For this review, take the finished solid that the model builds, in its own axes (mm). Face numbers are marked on the shaded views. A direction names the side the tool comes from. Give positions to 0.01 mm unless a question says otherwise; leave off trailing zeros. Loops run counter-clockwise (first coordinate to the right, second up) from the corner with the lowest first, then second, coordinate; pieces in that order, holes last. Notation, with made-up numbers: (35.5, -12) - (46.5, -12) arc R10 ccw to (46.5, -1) - close; hole circle Ø5 at (-25, -28). An arc over 180 degrees is marked (long way). Put each result on its own line as item: value.
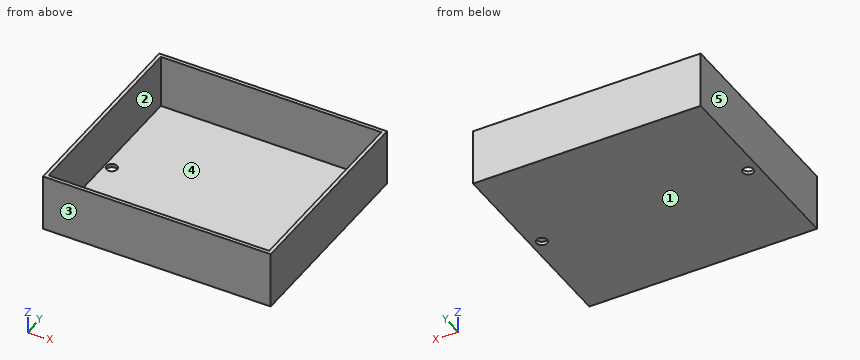
from build123d import *

# Parameters (mm, degrees)
SKETCH001_W     = 64
SKETCH001_H     = 57.5
PAD_DEPTH       = 16
SKETCH003_W     = 62
SKETCH003_H     = 55.5
POCKET001_DEPTH = 15
SKETCH002_R     = 1.5
POCKET_DEPTH    = 16.001


with BuildPart() as part:
    # Sketch001 → Pad (new body)
    with BuildSketch(Plane.XY):
        Rectangle(SKETCH001_W, SKETCH001_H)
    extrude(amount=PAD_DEPTH)

    # Sketch003 (on Face6 of Pad) → Pocket001 (cut)
    with BuildSketch(Plane.XY.offset(16)):
        Rectangle(SKETCH003_W, SKETCH003_H)
    extrude(amount=-POCKET001_DEPTH, mode=Mode.SUBTRACT)

    # Sketch002 (on Face6 of Pad) → Pocket (cut, through all)
    with BuildSketch(Plane.XY.offset(16)):
        with Locations((-29, 0)):
            Circle(SKETCH002_R)
        with Locations((29, 0)):
            Circle(SKETCH002_R)
    extrude(amount=-POCKET_DEPTH, mode=Mode.SUBTRACT)


solid = part.part
1) Insertion check: pin 1 Ø1.8 at (x, y) = (-29, 0) entering from +Z; pin 2 Ø1.5 at (x, y) = (20.5, -23) entering from +Z; pin 3 Ø3.5 at (x, y) = (29, 0) entering from -Z. Each pin has a flat end and moves straight along its axis. Give the tip position at first contact, or say it passes through.
Geometry check:
pin 1: passes through
pin 2: stops at z = 1
pin 3: stops at z = 0
2) Take a section at A-A on y = 0. State the section outline as (x, z) points.
Geometry check:
outline: (-32, 0) - (-30.5, 0) - (-30.5, 1) - (-31, 1) - (-31, 16) - (-32, 16) - close; (-27.5, 0) - (27.5, 0) - (27.5, 1) - (-27.5, 1) - close; (30.5, 0) - (32, 0) - (32, 16) - (31, 16) - (31, 1) - (30.5, 1) - close
3) Draft analysis for pull direction Y (two halves, no side actions). For the marked faces 1, 2 and 3, state which applies: pulls with the +Y half, pulls with the -Y half, needs draft (parallel to the pull), parting line crosses it, or undercut.
Geometry check:
face 1: needs draft
face 2: undercut
face 3: pulls with the -Y half
4) For the marked faces 4 and 5, list the 3-axis set-ups (+Z, -Z, +X, -X, +Y, -Y) from which the entire face can be reached by the end or side of a thin tool; tool diameter is ignored.
Geometry check:
face 4: +Z
face 5: +Z, -Z, -X, +Y, -Y
5) Take a section at B-B on x = -29. State the section outline as (y, z) points, and give its area (3 significant figures).
Geometry check:
outline: (-28.75, 0) - (-1.5, 0) - (-1.5, 1) - (-27.75, 1) - (-27.75, 16) - (-28.75, 16) - close; (1.5, 0) - (28.75, 0) - (28.75, 16) - (27.75, 16) - (27.75, 1) - (1.5, 1) - close
area: 84.5 mm²
6) Take a section at D-D on y = 18.5. State the section outline as (x, z) points, and give its area (3 significant figures).
Geometry check:
outline: (-32, 0) - (32, 0) - (32, 16) - (31, 16) - (31, 1) - (-31, 1) - (-31, 16) - (-32, 16) - close
area: 94.0 mm²
7) Take a section at C-C on z = 2.5. State the section outline as (x, y) points.
Geometry check:
outline: (-32, -28.75) - (32, -28.75) - (32, 28.75) - (-32, 28.75) - close; hole (-31, -27.75) - (31, -27.75) - (31, 27.75) - (-31, 27.75) - close
8) Wall thickness on line 1 (Y direction, x = -15, z = 12.5); line 2 (Y direction, x = 29, z = 0.85); line 3 (X direction, y = 11, z = 10): over which ranges is each line inside the solid? List them lowest first.
Geometry check:
line 1: y = -28.75 to -27.75, 27.75 to 28.75
line 2: y = -28.75 to -1.5, 1.5 to 28.75
line 3: x = -32 to -31, 31 to 32
